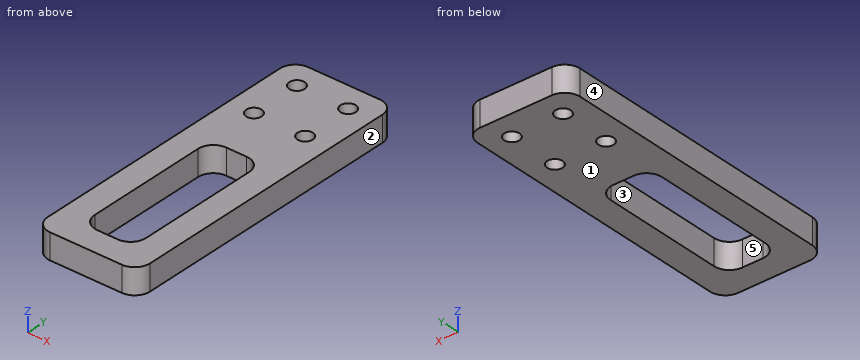
```python
from build123d import *

# Parameters (mm, degrees)
SKETCH_1_W          = 20
SKETCH_1_H          = 60
EXTRUDE_1_DEPTH     = 5
SKETCH_2_R          = 1.5
CUT_EXTRUDE_1_DEPTH = 33.015621187
SKETCH_3_W          = 10
SKETCH_3_H          = 30
CUT_EXTRUDE_2_DEPTH = 33.015621187
FILLET_1_R          = 3


with BuildPart() as part:
    # 草图1 → 凸台-拉伸1 (new body)
    with BuildSketch(Plane.XY):
        Rectangle(SKETCH_1_W, SKETCH_1_H)
    extrude(amount=EXTRUDE_1_DEPTH)

    # 草图2 → 切除-拉伸1 (cut, through all)
    with BuildSketch(Plane.XY.offset(5)):
        with Locations((-5, 25)):
            Circle(SKETCH_2_R)
        with Locations((-5, 15)):
            Circle(SKETCH_2_R)
        with Locations(Location((5, 15, 0), (0, 0, 180))):
            Circle(SKETCH_2_R)
        with Locations(Location((5, 25, 0), (0, 0, 180))):
            Circle(SKETCH_2_R)
    extrude(amount=-CUT_EXTRUDE_1_DEPTH, mode=Mode.SUBTRACT)

    # 草图3 → 切除-拉伸2 (cut, through all)
    with BuildSketch(Plane.XY.offset(5)):
        with Locations((0, -10)):
            Rectangle(SKETCH_3_W, SKETCH_3_H)
    extrude(amount=-CUT_EXTRUDE_2_DEPTH, mode=Mode.SUBTRACT)

    # 圆角1
    fillet_1_edges = [part.edges().sort_by_distance(p)[0] for p in [
        (5, 5, 2.5),
        (5, -25, 2.5),
        (-5, -25, 2.5),
        (-5, 5, 2.5),
        (10, -30, 2.5),
        (-10, -30, 2.5),
        (-10, 30, 2.5),
        (10, 30, 2.5),
    ]]
    fillet(fillet_1_edges, radius=FILLET_1_R)


solid = part.part
```
Build history of the part. All positions in model axes, mm. Face numbers are marked on the shaded views. A direction names the side the tool comes from. Round coordinates to 2 decimals unless told otherwise and drop trailing zeros. Order: outer loops, then holes, each group sorted by start corner. A loop starts at its lowest first (then second) coordinate and runs counter-clockwise, first axis right, second up. Notation, with made-up numbers: (22, 55) - (53, 55) arc R25 ccw to (53, 68) - close; hole circle Ø8 at (5.25, 72). An arc over 180 degrees is marked (long way). Use a Markdown table: item, result.
1) Pull direction X, two halves, no side cores. Call the marked faces 1, 2 and 3: pulls with the +X half, pulls with the -X half, needs draft (parallel to the pull), parting line crosses it, or undercut.
Recorded:
| item | result |
|---|---|
| face 1 | needs draft |
| face 2 | pulls with the +X half |
| face 3 | undercut |
2) Tool access for the marked faces 4 and 5: list every direction of +Z, -Z, +X, -X, +Y, -Y with a clear straight run to the whole face (end or side of a thin tool).
Recorded:
| item | result |
|---|---|
| face 4 | +Z, -Z, -X, +Y, -Y |
| face 5 | +Z, -Z |
3) Saw through at C-C on x = -4.25. Write the cut outline in (y, z), and give its area (3 significant figures).
Recorded:
| item | result |
|---|---|
| outline | (-30, 0) - (-23.98, 0) - (-23.98, 5) - (-30, 5) - close; (3.98, 0) - (13.7, 0) - (13.7, 5) - (3.98, 5) - close; (16.3, 0) - (23.7, 0) - (23.7, 5) - (16.3, 5) - close; (26.3, 0) - (30, 0) - (30, 5) - (26.3, 5) - close |
| area | 134 mm² |
4) Saw through at B-B on z = 0.65. Write the cut outline in (x, y).
Recorded:
| item | result |
|---|---|
| outline | (-10, -27) arc R3 ccw to (-7, -30) - (7, -30) arc R3 ccw to (10, -27) - (10, 27) arc R3 ccw to (7, 30) - (-7, 30) arc R3 ccw to (-10, 27) - close; hole circle Ø3 at (-5, 15); hole circle Ø3 at (-5, 25); hole (-5, -22) arc R3 ccw to (-2, -25) - (2, -25) arc R3 ccw to (5, -22) - (5, 2) arc R3 ccw to (2, 5) - (-2, 5) arc R3 ccw to (-5, 2) - close; hole circle Ø3 at (5, 15); hole circle Ø3 at (5, 25) |
5) Saw through at A-A on y = 15. Write the cut outline in (x, z).
Recorded:
| item | result |
|---|---|
| outline | (-10, 0) - (-6.5, 0) - (-6.5, 5) - (-10, 5) - close; (-3.5, 0) - (3.5, 0) - (3.5, 5) - (-3.5, 5) - close; (6.5, 0) - (10, 0) - (10, 5) - (6.5, 5) - close |
6) Saw through at D-D on y = -17.5. Write the cut outline in (x, z), and give its area (3 significant figures).
Recorded:
| item | result |
|---|---|
| outline | (-10, 0) - (-5, 0) - (-5, 5) - (-10, 5) - close; (5, 0) - (10, 0) - (10, 5) - (5, 5) - close |
| area | 50.0 mm² |
7) Wall check: L1, parallel to X at y = -15.5, z = 1.5; L2, parallel to Y at x = 0.5, z = 2.15; L3, parallel to Y at x = 3.75, z = 3. Give the ranges that are in metal, low to high.
Recorded:
| item | result |
|---|---|
| L1 | x = -10 to -5, 5 to 10 |
| L2 | y = -30 to -25, 5 to 30 |
| L3 | y = -30 to -24.44, 4.44 to 14.17, 15.83 to 24.17, 25.83 to 30 |
